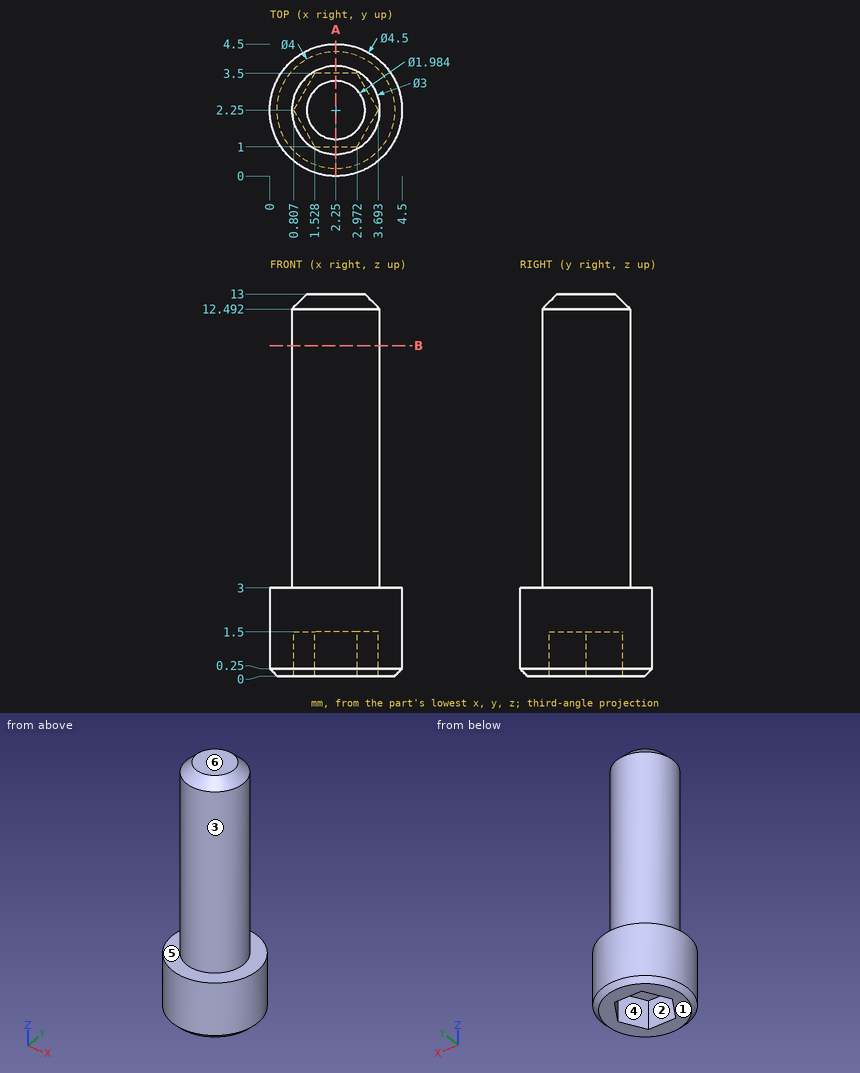
Geometry check sheet. Reference: drawing and pictorial views, mm from the part's lowest x, y, z. A direction names the side the tool comes from. Round coordinates to 2 decimals unless told otherwise and drop trailing zeros. Order: outer loops, then holes, each group sorted by start corner. A loop starts at its lowest first (then second) coordinate and runs counter-clockwise, first axis right, second up. Notation, with made-up numbers: (55, 88.5) - (96, 88.5) arc R19 cw to (96, 118.5) - close; hole circle Ø10 at (-19, -22). An arc over 180 degrees is marked (long way). One line per question, with ' | ' between items. Start each with the question number.
(1) Access from +Z, -Z, +X, -X, +Y, -Y to the whole of each face (thin tool, end or side, straight path). Record for the marked faces 5 and 6.
(2) Sectioned sample at B-B on z = 11.25. Record the cut outline in (x, y).
(3) Thickness scan on L1, parallel to Z at x = 2.25, y = 2.05; L2, parallel to Z at x = 2.15, y = 3.85; L3, parallel to X at y = 2.2, z = 12.25. Record the ranges inside material, lowest first. Write a range as [from, to].
(4) Sectioned sample at A-A on x = 2.25. Record the cut outline in (y, z).
(5) Release check for a two-part mould opening along X. For the marked faces 1, 2, 3 and 4 record: released by +X, released by -X, zero draft, split by the parting line, or undercut.
Conclusion:
1) face 5: +Z | face 6: +Z, +X, -X, +Y, -Y
2) outline: circle Ø3 at (2.25, 2.25)
3) L1: z = [1.5, 13] | L2: z = [0, 3] | L3: x = [0.75, 3.75]
4) outline: (0, 0.25) - (0.25, 0) - (1, 0) - (1, 1.5) - (3.5, 1.5) - (3.5, 0) - (4.25, 0) - (4.5, 0.25) - (4.5, 3) - (3.75, 3) - (3.75, 12.49) - (3.24, 13) - (1.26, 13) - (0.75, 12.49) - (0.75, 3) - (0, 3) - close
5) face 1: zero draft | face 2: undercut | face 3: split by the parting line | face 4: undercut
